Geometry check sheet. Reference: the model listing, model coordinates, mm. A direction names the side the tool comes from. Give positions to 0.01 mm unless a question says otherwise; leave off trailing zeros. Write each loop counter-clockwise with the first axis right and the second up, starting at its lowest first coordinate (ties: lowest second). Pieces come first, ordered by that corner, then holes. Notation, with made-up numbers: (87, 4.25) -> (144, 4.25) arc R11 cw to (144, 17.25) -> close; hole circle Ø6 at (51.5, -20). An arc over 180 degrees is marked (long way). Write item = value, one per line. Start each with the question number.
1. Thickness scan on line 1 along Z through (x, y) = (3, 9); line 2 along X through (y, z) = (11, 20.25); line 3 along Y through (x, z) = (1.5, 4.5). Record the ranges inside material, lowest first.
2. Mould release check, pull along Z, two halves, no side actions. Record for faces 3 (the cylindrical face through (1.714, 12.699, 24.715)), 4 (the flat face through (2, 13, 12)), 5 (the flat face through (2, 12, 4)): pulls with the +Z half, pulls with the -Z half, needs draft (parallel to the pull), parting line crosses it, or undercut.
3. Cross-section at B-B, the plane z = 4.5. Record the cut outline in (x, y), plus the area to 3 significant figures.
4. Cross-section at A-A, the plane x = 2. Record the cut outline in (y, z), plus the area to 3 significant figures.
5. Cross-section at C-C, the plane y = 9. State how many separate pieces and enclosed holes the cut face has, plus the area to 3 significant figures.
6. Set-up check for faces 1 (the cylindrical face through (1.714, 12.715, 0.301)), 2 (the flat face through (2, 6, 3.788)): record each of +Z, -Z, +X, -X, +Y, -Y from which the full face is reachable in a straight line by a thin tool's end or side.
7. Cross-section at D-D, the plane z = 14.75. Record the cut outline in (x, y), plus the area to 3 significant figures.
8. Depth check by flat-ended pin: P1, Ø1.1, axis at y = 5.5, z = 4.5, coming from the -X side; P2, Ø3, axis at y = 11, z = 15, coming from the -X side; P3, Ø0.7, axis at x = 1, z = 4.5, coming from the -Y side. Enter the tip coordinate at first touch or a pass-through.
Autodesk Inventor part; units mm, degrees
ref_plane "YZ Plane" through (0, 0, 0) normal (1, 0, 0) x (0, 1, 0)
ref_plane "XZ Plane" through (0, 0, 0) normal (0, 1, 0) x (-1, 0, 0)
ref_plane "XY Plane" through (0, 0, 0) normal (0, 0, 1) x (1, 0, 0)
sketch "Sketch1" plane through (0, 0, 0) normal (0, 0, 1) x (1, 0, 0)
  line L0 (-4.7637, 0) -> (8.2363, 0)
  line L1 (8.2363, 0) -> (8.2363, 13)
  line L2 (8.2363, 13) -> (-4.7637, 13)
  line L3 (-4.7637, 13) -> (-4.7637, 0)
  arc A0 (-4.7637, 0) -> (-0.7637, 13) centre (-33.6274, 15.9965) ccw
  arc A1 (4.2363, 13) -> (8.2363, 0) centre (37.1, 15.9965) ccw
  point P0 (0, 0)
  dimension "d0" = 13
  dimension "d1" = 13
  dimension "d2" = 4
  dimension "d3" = 4
  dimension "d4" = 33
  dimension "d5" = 33
extrude "Extrusion1" add sketch "Sketch1" along normal blind 25 contours A0 L2 A1 L0
sketch "Sketch2" plane through (-4.7637, 0, 0) normal (0, -1, 0) x (1, 0, 0)
  line L0 (4, 21.2125) -> (9.2, 21.2125)
  line L1 (9.2, 21.2125) -> (9.2, 19.8125)
  line L2 (9.2, 19.8125) -> (4, 19.8125)
  line L3 (4, 19.8125) -> (4, 21.2125)
  line L4 (4, 5.1875) -> (9.2, 5.1875)
  line L5 (9.2, 5.1875) -> (9.2, 3.7875)
  line L6 (9.2, 3.7875) -> (4, 3.7875)
  line L7 (4, 3.7875) -> (4, 5.1875)
  line L8 (0, 0) -> (0, 25)
  line L9 (0, 25) -> (13, 25)
  point P0 (4.7637, 0)
  dimension "d8" = 5.2
  dimension "d9" = 4
  dimension "d10" = 1.4
  dimension "d11" = 1.4
  dimension "d12" = 17.425
  dimension "d13" = 3.7875
extrude "Extrusion2" cut sketch "Sketch2" against normal blind 2
sketch "Sketch3" plane through (-4.7637, 2, 0) normal (0, -1, 0) x (1, 0, 0)
  line L0 (4.4, 21.2125) -> (8.8, 21.2125)
  line L1 (8.8, 21.2125) -> (8.8, 19.8125)
  line L2 (8.8, 19.8125) -> (4.4, 19.8125)
  line L3 (4.4, 19.8125) -> (4.4, 21.2125)
  line L4 (4, 19.8125) -> (4, 21.2125)
  line L5 (9.2, 21.2125) -> (9.2, 19.8125)
  line L6 (4, 21.2125) -> (9.2, 21.2125)
  line L7 (9.2, 19.8125) -> (4, 19.8125)
  line L8 (4, 5.1875) -> (9.2, 5.1875)
  line L9 (4, 3.7875) -> (4, 5.1875)
  line L10 (9.2, 3.7875) -> (4, 3.7875)
  line L11 (9.2, 5.1875) -> (9.2, 3.7875)
  line L12 (9.2, 3.7875) -> (4, 3.7875)
  line L13 (4.4, 5.1875) -> (8.8, 5.1875)
  line L14 (8.8, 5.1875) -> (8.8, 3.7875)
  line L15 (8.8, 3.7875) -> (4.4, 3.7875)
  line L16 (4.4, 3.7875) -> (4.4, 5.1875)
  point P0 (4.7637, 0)
  dimension "d16" = 0.4
  dimension "d17" = 0.4
  dimension "d18" = 0
  dimension "d19" = 0
extrude "Extrusion3" cut sketch "Sketch3" against normal blind 10 contours L0 L1 L2 L3 | L8 L14 L10 L16
fillet "Fillet1" radius 1 8 edges at (4.2363, 13, 12.5) (1.7363, 13, 25) (-0.7637, 13, 12.5) (1.7363, 13, 0) (5.5593, 6.2917, 25) (-2.0867, 6.2917, 25) (5.5593, 6.2917, 0) (-2.0867, 6.2917, 0)
properties part number "DoubleSliderCap-wide"
Answers:
q1.line_1 = 0 to 3.79, 5.19 to 19.81, 21.21 to 25
q1.line_2 = -1.01 to -0.36, 4.04 to 4.48
q1.line_3 = 12 to 13
q2.face_3 = pulls with the +Z half
q2.face_4 = needs draft
q2.face_5 = undercut
q3.outline = (-4.76, 0) -> (-0.76, 0) -> (-0.76, 2) -> (-0.36, 2) -> (-0.36, 12) -> (4.04, 12) -> (4.04, 2) -> (4.44, 2) -> (4.44, 0) -> (8.24, 0) arc R33 cw to (4.33, 12.12) arc R1 ccw to (3.34, 13) -> (0.14, 13) arc R1 ccw to (-0.86, 12.12) arc R33 cw to start
q3.area = 49.4 mm^2
q4.outline = (0, 0) -> (12, 0) arc R1 ccw to (13, 1) -> (13, 24) arc R1 ccw to (12, 25) -> (0, 25) -> (0, 21.21) -> (12, 21.21) -> (12, 19.81) -> (0, 19.81) -> (0, 5.19) -> (12, 5.19) -> (12, 3.79) -> (0, 3.79) -> close
q4.area = 291 mm^2
q5.separate_pieces = 1
q5.enclosed_holes = 2
q5.area = 142 mm^2
q6.face_1 = -Z, +X, -X, +Y
q6.face_2 = -Y
q7.outline = (-4.76, 0) -> (8.24, 0) arc R33 cw to (4.33, 12.12) arc R1 ccw to (3.34, 13) -> (0.14, 13) arc R1 ccw to (-0.86, 12.12) arc R33 cw to start
q7.area = 104 mm^2
q8.P1 = -2.53
q8.P2 = -1.27
q8.P3 = 12
